The listing builds one solid part. Answer for the finished solid, in the listing's coordinates (mm). Face numbers are marked on the shaded views. A direction names the side the tool comes from. Round coordinates to 2 decimals unless told otherwise and drop trailing zeros. Loops run counter-clockwise (first coordinate to the right, second up) from the corner with the lowest first, then second, coordinate; pieces in that order, holes last. Notation, with made-up numbers: (68.5, 57.5) - (110.5, 57.5) arc R22 ccw to (110.5, 83.5) - close; hole circle Ø4 at (61, 51.25). An arc over 180 degrees is marked (long way). One line per item, written item: value.
```python
from build123d import *

# Parameters (mm, degrees)
BOSS_EXTRUDE1_DEPTH                = 6
BOSS_EXTRUDE2_DEPTH                = 4
M1_2X0_25_TAPPED_HOLE1_D           = 0.95
M1_2X0_25_TAPPED_HOLE1_DEPTH       = 3.15
M1_2X0_25_TAPPED_HOLE1_CBORE_D     = 1.2
M1_2X0_25_TAPPED_HOLE1_CBORE_DEPTH = 2.4
M1_2X0_25_TAPPED_HOLE1_TIP         = 0.285408794


with BuildPart() as part:
    # Sketch2 → Boss-Extrude1 (new body)
    with BuildSketch(Plane.XY):
        with BuildLine():
            Line((-131.1, -7.893462557), (-131.1, -5))
            Line((-131.1, -5), (-133.4, -5))
            Line((-133.4, -5), (-133.4, -7.893462557))
            ThreePointArc((-133.4, -7.893462557), (-133.839435478, -8.201752281), (-134.199358869, -8.6))
            Line((-134.199358869, -8.6), (-137.15, -8.6))
            Line((-137.15, -8.6), (-137.15, -11.4))
            Line((-137.15, -11.4), (-134.199358869, -11.4))
            ThreePointArc((-134.199358869, -11.4), (-132.25, -12.4), (-130.300641131, -11.4))
            Line((-130.300641131, -11.4), (-127.35, -11.4))
            Line((-127.35, -11.4), (-127.35, -8.6))
            Line((-127.35, -8.6), (-130.300641131, -8.6))
            ThreePointArc((-130.300641131, -8.6), (-130.660564522, -8.201752281), (-131.1, -7.893462557))
        make_face()
    extrude(amount=-BOSS_EXTRUDE1_DEPTH)

    # Sketch3 → Boss-Extrude2 (add)
    with BuildSketch(Plane(origin=(0, -5, 0), x_dir=(1, 0, 0), z_dir=(0, 1, 0))):
        with BuildLine():
            ThreePointArc((-133.4, 1.15), (-132.25, 0), (-131.1, 1.15))
            Line((-131.1, 1.15), (-133.4, 1.15))
        make_face()
        with BuildLine():
            Line((-133.4, 1.15), (-131.1, 1.15))
            ThreePointArc((-131.1, 1.15), (-132.25, 2.3), (-133.4, 1.15))
        make_face()
    extrude(amount=BOSS_EXTRUDE2_DEPTH)

    # M1.2x0.25 Tapped Hole1
    with Locations(Plane(origin=(-132.25, -1, -1.15), x_dir=(0, 0, 1), z_dir=(0, 1, 0))):
        with Locations((0, 0)):
            CounterBoreHole(M1_2X0_25_TAPPED_HOLE1_D / 2, M1_2X0_25_TAPPED_HOLE1_CBORE_D / 2, M1_2X0_25_TAPPED_HOLE1_CBORE_DEPTH, depth=M1_2X0_25_TAPPED_HOLE1_DEPTH)
            with Locations((0, 0, -(M1_2X0_25_TAPPED_HOLE1_DEPTH + M1_2X0_25_TAPPED_HOLE1_TIP / 2))):  # 118° drill point
                Cone(0, M1_2X0_25_TAPPED_HOLE1_D / 2, M1_2X0_25_TAPPED_HOLE1_TIP, mode=Mode.SUBTRACT)


solid = part.part
```
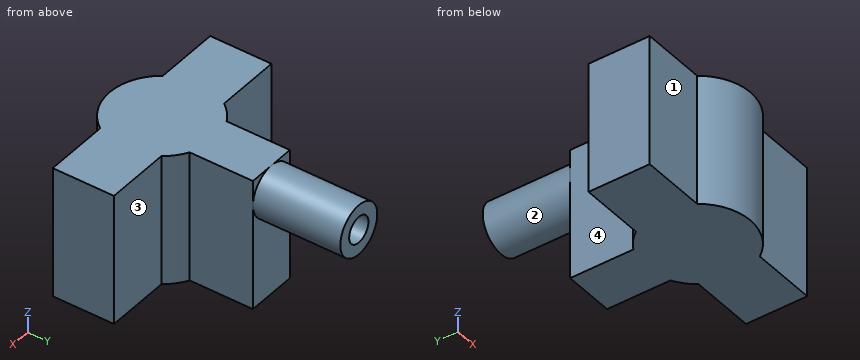
1) For the marked faces 1, 2, 3 and 4, determine the directions among +Z, -Z, +X, -X, +Y, -Y from which every point of the face is accessible in a straight line to the end or side of a thin tool.
Final values:
face 1: +Z, -Z, -X, -Y
face 2: +Y
face 3: +Z, -Z, +X, +Y
face 4: +Z, -Z, -X, +Y
2) Each of these flat-tipped pins is pushed along its axis until it touches: pin 1 Ø3 at (x, y) = (-131.5, -8) entering from +Z; pin 2 Ø0.9 at (x, z) = (-135.5, -2.5) entering from +Y; pin 3 Ø0.7 at (x, z) = (-132.5, -4) entering from +Y; pin 4 Ø2.5 at (y, z) = (-6, -3) entering from +X. Where does it stop, or does it pass through?
Final values:
pin 1: z = 0
pin 2: y = -8.6
pin 3: y = -5
pin 4: x = -131.1
3) Consider L1, parallel to Z at x = -132.25, y = -3.85 (3 decimals); L2, parallel to Z at x = -132.25, y = -1.95; L3, parallel to X at y = -3.65, z = -1.15 (3 decimals). Determine where each line is inside the solid, lowest interval first.
Final values:
L1: -2.3 to -1.625, -0.675 to 0
L2: -2.3 to -1.75, -0.55 to 0
L3: -133.4 to -132.725, -131.775 to -131.1
4) A cutting plane is placed at A-A on z = -4. Give the vertices of the cut face in (x, y), and give its area (3 significant figures).
Final values:
outline: (-137.15, -11.4) - (-134.2, -11.4) arc R2.4 ccw to (-130.3, -11.4) - (-127.35, -11.4) - (-127.35, -8.6) - (-130.3, -8.6) arc R2.4 ccw to (-131.1, -7.89) - (-131.1, -5) - (-133.4, -5) - (-133.4, -7.89) arc R2.4 ccw to (-134.2, -8.6) - (-137.15, -8.6) - close
area: 39.1 mm2
5) A cutting plane is placed at C-C on x = -129.75. Give the vertices of the cut face in (y, z), and give its area (3 significant figures).
Final values:
outline: (-11.4, -6) - (-8.6, -6) - (-8.6, 0) - (-11.4, 0) - close
area: 16.8 mm2
6) A cutting plane is placed at B-B on y = -6.25. Give the vertices of the cut face in (x, z), and give its area (3 significant figures).
Final values:
outline: (-133.4, -6) - (-131.1, -6) - (-131.1, 0) - (-133.4, 0) - close
area: 13.8 mm2
